Source: three-view drawing plus pictorial views. Frame: mm from the lowest corner of the part. Give positions to 0.01 mm unless a question says otherwise; leave off trailing zeros. Order: outer loops, then holes, each group sorted by start corner. A loop starts at its lowest first (then second) coordinate and runs counter-clockwise, first axis right, second up. Notation, with made-up numbers: M 4,77.25 L 30,77.25 A18 ccw 30,85.25 Z; hole C 29.5,-14 d5. An arc over 180 degrees is marked long. One line per item, written item: value. Start each with the question number.
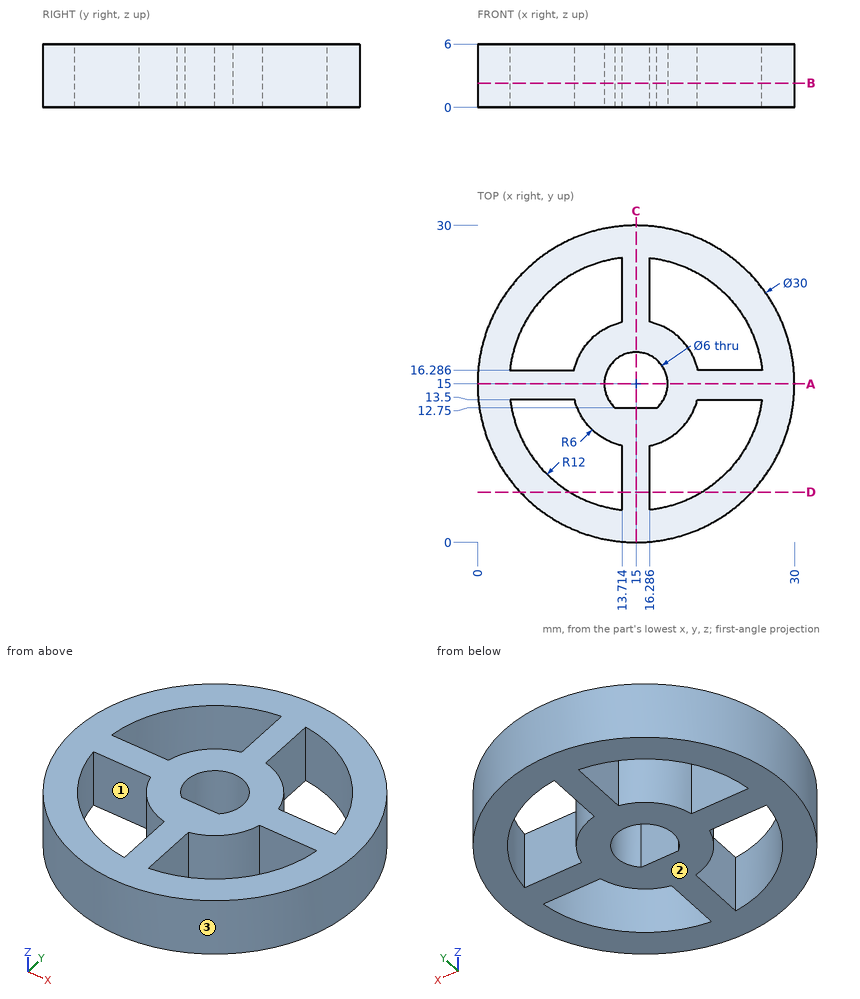
Q1. Section query B-B on z = 2.3. Return loops of the section in (x, y), and give its area (3 significant figures).
Q2. Section query D-D on y = 4.75. Return loops of the section in (x, z).
Q3. Mould query, pull axis Y, two halves, no side actions, for the marked faces 1, 2 and 3. Classes: +Y half, -Y half, draft (parallel to the pull), parting line (faces both ways), or undercut.
Q4. Section query A-A on y = 15. Return loops of the section in (x, z).
Q5. Section query C-C on x = 15. Return loops of the section in (y, z), and give its area (4 significant figures).
Q6. Ray query, line 1 along Y through (x, z) = (15, 4); line 2 along Y through (x, z) = (23, 2.85) (1 decimal); line 3 along Y through (x, z) = (18.75, 2.1) (1 decimal). Return the intervals inside material, ascending. Write a range as [from, to].
Q7. Contact query for flat-ended pins moving along their axis: pin 1 (3 mm diameter, centred on y = 7, z = 4.5, fed in from +X); pin 2 (3 mm diameter, centred on y = 7, z = 3.5, fed in from -X); pin 3 (2 mm diameter, centred on x = 6, z = 1, fed in from +Y); pin 4 (9.5 mm diameter, centred on x = 15, y = 15, fed in from -Z). Output: stop coordinate, or through.
Results below:
1. outline: C 15,15 d30; hole M 3.07,16.29 L 9.14,16.29 A6 cw 13.71,20.86 L 13.71,26.93 A12 ccw Z; hole M 3.09,13.5 A12 ccw 13.71,3.07 L 13.71,9.14 A6 cw 9.19,13.5 Z; hole M 13.02,12.75 L 16.98,12.75 A3 ccw long Z; hole M 16.29,3.07 A12 ccw 26.91,13.5 L 20.81,13.5 A6 cw 16.29,9.14 Z; hole M 16.29,20.86 A6 cw 20.86,16.29 L 26.93,16.29 A12 ccw 16.29,26.93 Z
1. area: 406 mm2
2. outline: M 4.05,0 L 8.76,0 L 8.76,6 L 4.05,6 Z; M 13.71,0 L 16.29,0 L 16.29,6 L 13.71,6 Z; M 21.24,0 L 25.95,0 L 25.95,6 L 21.24,6 Z
3. face 1: undercut
3. face 2: draft
3. face 3: parting line
4. outline: M 0,0 L 12,0 L 12,6 L 0,6 Z; M 18,0 L 30,0 L 30,6 L 18,6 Z
5. outline: M 0,0 L 12.75,0 L 12.75,6 L 0,6 Z; M 18,0 L 30,0 L 30,6 L 18,6 Z
5. area: 148.5 mm2
6. line 1: [0, 12.75], [18, 30]
6. line 2: [2.3, 6.1], [13.5, 16.3], [23.9, 27.7]
6. line 3: [0.5, 3.6], [10.3, 19.7], [26.4, 29.5]
7. pin 1: x = 28.52
7. pin 2: x = 1.48
7. pin 3: y = 27.69
7. pin 4: z = 0
